from build123d import *

# Parameters (mm, degrees)
SKETCH_1_R          = 20
SKETCH_1_R_2        = 4
SKETCH_1_R_3        = 0.65
EXTRUDE_1_DEPTH     = 5.5
CUT_EXTRUDE_START   = -3.5
CUT_EXTRUDE_1_DEPTH = 3.5
SKETCH_3_R          = 1.5
CUT_EXTRUDE_2_DEPTH = 13
CHAMFER_1_SIZE      = 0.5
CHAMFER_2_SIZE      = 0.5


with BuildPart() as part:
    # 草图1 → 凸台-拉伸1 (new body)
    with BuildSketch(Plane.XY):
        Circle(SKETCH_1_R)
        Circle(SKETCH_1_R_2, mode=Mode.SUBTRACT)
        with Locations((6, 0)):
            Circle(SKETCH_1_R_3, mode=Mode.SUBTRACT)
        with Locations((8.5, 0)):
            Circle(SKETCH_1_R_3, mode=Mode.SUBTRACT)
        with Locations((11, 0)):
            Circle(SKETCH_1_R_3, mode=Mode.SUBTRACT)
        with Locations((13.5, 0)):
            Circle(SKETCH_1_R_3, mode=Mode.SUBTRACT)
        with Locations((16, 0)):
            Circle(SKETCH_1_R_3, mode=Mode.SUBTRACT)
        with Locations(Location((-16, 0, 0), (0, 0, 180))):
            Circle(SKETCH_1_R_3, mode=Mode.SUBTRACT)
        with Locations(Location((-13.5, 0, 0), (0, 0, 180))):
            Circle(SKETCH_1_R_3, mode=Mode.SUBTRACT)
        with Locations(Location((-11, 0, 0), (0, 0, 180))):
            Circle(SKETCH_1_R_3, mode=Mode.SUBTRACT)
        with Locations(Location((-8.5, 0, 0), (0, 0, 180))):
            Circle(SKETCH_1_R_3, mode=Mode.SUBTRACT)
        with Locations(Location((-6, 0, 0), (0, 0, 180))):
            Circle(SKETCH_1_R_3, mode=Mode.SUBTRACT)
    extrude(amount=EXTRUDE_1_DEPTH)

    # 草图2 → 切除-拉伸1 (cut)
    with BuildSketch(Plane.XY.offset(5.5).offset(CUT_EXTRUDE_START)):
        with BuildLine():
            Line((-16.234375, 2.488989425), (-0.375, 3.982383081))
            ThreePointArc((-0.375, 3.982383081), (0, 4), (0.375, 3.982383081))
            Line((0.375, 3.982383081), (16.234375, 2.488989425))
            ThreePointArc((16.234375, 2.488989425), (18.5, 0), (16.234375, -2.488989425))
            Line((16.234375, -2.488989425), (0.375, -3.982383081))
            ThreePointArc((0.375, -3.982383081), (0, -4), (-0.375, -3.982383081))
            Line((-0.375, -3.982383081), (-16.234375, -2.488989425))
            ThreePointArc((-16.234375, -2.488989425), (-18.5, 0), (-16.234375, 2.488989425))
        make_face()
    extrude(amount=CUT_EXTRUDE_1_DEPTH, mode=Mode.SUBTRACT)

    # 草图3 → 切除-拉伸2 (cut)
    with BuildSketch(Plane.XY.offset(5.5)):
        with Locations((0, 16)):
            Circle(SKETCH_3_R)
        with Locations((13.856406461, -8)):
            Circle(SKETCH_3_R)
        with Locations((-13.856406461, -8)):
            Circle(SKETCH_3_R)
    extrude(amount=-CUT_EXTRUDE_2_DEPTH, mode=Mode.SUBTRACT)

    # 倒角1
    chamfer_1_edges = [part.edges().sort_by_distance(p)[0] for p in [
        (-20, 0, 5.5),
    ]]
    chamfer(chamfer_1_edges, length=CHAMFER_1_SIZE)

    # 倒角2
    chamfer_2_edges = [part.edges().sort_by_distance(p)[0] for p in [
        (0, 4, 5.5),
        (0, -4, 5.5),
        (-8.3046875, 3.235686253, 5.5),
        (-18.5, 0, 5.5),
        (-8.3046875, -3.235686253, 5.5),
        (8.3046875, -3.235686253, 5.5),
        (18.5, 0, 5.5),
        (8.3046875, 3.235686253, 5.5),
    ]]
    chamfer(chamfer_2_edges, length=CHAMFER_2_SIZE)


solid = part.part
Read the model definition and answer for the solid it produces. Units are mm, in the model's axes. A direction names the side the tool comes from. Round coordinates to 2 decimals unless told otherwise and drop trailing zeros. Order: outer loops, then holes, each group sorted by start corner. A loop starts at its lowest first (then second) coordinate and runs counter-clockwise, first axis right, second up.
1) The part is cut by section A-A on z = 3.9. Write down the section's boundary in (x, y) (3 decimals), plus the area to 3 significant figures.
2) The mould has two halves that part along X. Classify faces 3 (the face through (4.2, 0.3, 0)), 4 (the face through (-15.35, -0.03, 0.99)), 5 (the face through (-4.336, -19.524, 2.465)): released by +X, released by -X, zero draft, split by the parting line, or undercut.
3) Flat-ended cylindrical pins translate along their axes: pin 1 (2 mm diameter, centred on x = -13.5, y = 0, fed in from +Z); pin 2 (1 mm diameter, centred on x = 16, y = 0, fed in from -Z); pin 3 (2 mm diameter, centred on y = 12.5, z = 4, fed in from +X); pin 4 (3 mm diameter, centred on y = -11.5, z = 4.5, fed in from -X). Find the tip coordinate at first contact, or state that the pin passes through.
4) The part is cut by section B-B on x = -13.5. Give the number of separate pieces and of enclosed holes in the cut face, plus the area to 3 significant figures.
5) Straight lines are drawn through the part: L1, parallel to Y at x = 0, z = 4.3; L2, parallel to Y at x = 14, z = 3.75; L3, parallel to X at y = -7, z = 4.9 (3 decimals). For each, find the intervals that lie inside material, in ascending order.
6) For faces 1 (the face through (6.62, 0.2, 0.99)), 2 (the face through (8.439, -3.471, 5.246)), determine the directions among +Z, -Z, +X, -X, +Y, -Y from which every point of the face is accessible in a straight line to the end or side of a thin tool.
Resolved:
1. outline: circle Ø40 at (0, 0); hole (-16.234, -2.489) - (-0.375, -3.982) arc R4 ccw to (0.375, -3.982) - (16.234, -2.489) arc R2.5 ccw to (16.234, 2.489) - (0.375, 3.982) arc R4 ccw to (-0.375, 3.982) - (-16.234, 2.489) arc R2.5 ccw to start; hole circle Ø3 at (-13.856, -8); hole circle Ø3 at (0, 16); hole circle Ø3 at (13.856, -8)
1. area: 1,010 mm2
2. face 3: zero draft
2. face 4: undercut
2. face 5: split by the parting line
3. pin 1: stops at z = 2
3. pin 2: passes through
3. pin 3: stops at x = 16.36
3. pin 4: stops at x = -17.32
4. separate pieces: 3
4. enclosed holes: 0
4. area: 124 mm2
5. L1: y = -20 to -4, 4 to 14.5, 17.5 to 20
5. L2: y = -14.28 to -9.49, -6.51 to -2.7, 2.7 to 14.28
5. L3: x = -18.735 to -14.974, -12.738 to 12.738, 14.974 to 18.735
6. face 1: +Z, -Z
6. face 2: +Z
